The listing builds one solid part. Answer for the finished solid, in the listing's coordinates (mm). Face numbers are marked on the shaded views. A direction names the side the tool comes from. Coordinates: 2 decimals unless noted, no trailing zeros. Loops run counter-clockwise (first coordinate to the right, second up) from the corner with the lowest first, then second, coordinate; pieces in that order, holes last. Notation, with made-up numbers: (72, -29.5) -> (86, -29.5) arc R27 cw to (86, -7.5) -> close; hole circle Ø6 at (14.5, -36). An arc over 180 degrees is marked (long way). Answer in a Markdown table with one row per item.
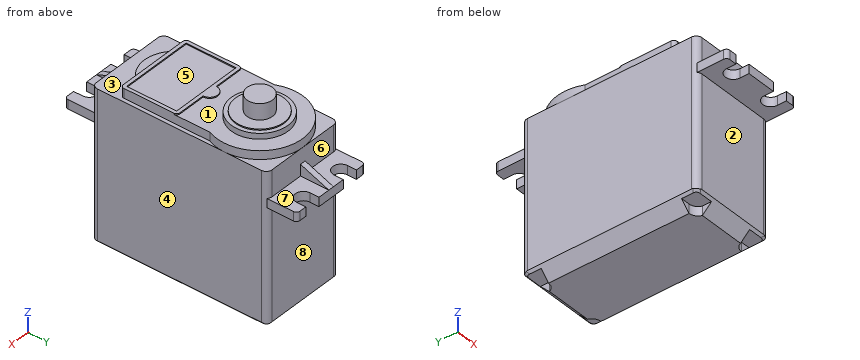
```python
from build123d import *

# Parameters (mm, degrees)
SKETCH1_W            = 35.433
SKETCH1_H            = 39.37
BOSS_EXTRUDE1_DEPTH  = 9.652
BOSS_EXTRUDE2_DEPTH  = 1.905
SKETCH3_R            = 6.35
BOSS_EXTRUDE3_DEPTH  = 1.27
SKETCH4_R            = 5.461
BOSS_EXTRUDE4_DEPTH  = 0.254
SKETCH6_R            = 2.8575
BOSS_EXTRUDE5_DEPTH  = 3.556
FILLET1_R            = 0.762
BOSS_EXTRUDE6_START  = 0.254
SKETCH7_W            = 16.129
SKETCH7_H            = 11.176
BOSS_EXTRUDE6_DEPTH  = 0.254
CHAMFER1_SIZE        = 2.54
FILLET3_R            = 1.27
FILLET4_R            = 1.27
CUT_EXTRUDE1_DEPTH   = 2.032
MIRROR2_COPY_1_DEPTH = 2.032
BOSS_EXTRUDE7_DEPTH  = 2.032
BOSS_EXTRUDE8_DEPTH  = 0.635


with BuildPart() as part:
    # Sketch1 → Boss-Extrude1 (new, symmetric)
    with BuildSketch(Plane(origin=(0, 0, 0), x_dir=(0, 0, -1), z_dir=(1, 0, 0))):
        Rectangle(SKETCH1_W, SKETCH1_H)
    extrude(amount=BOSS_EXTRUDE1_DEPTH, both=True)

    # Sketch2 → Boss-Extrude2 (add)
    with BuildSketch(Plane.XY.offset(17.7165)):
        with BuildLine():
            Line((-8.8265, 6.127362824), (-8.8265, -13.8938))
            Line((-8.8265, -13.8938), (-4.7625, -13.8938))
            ThreePointArc((-4.7625, -13.8938), (0, -15.817151304), (4.7625, -13.8938))
            Line((4.7625, -13.8938), (8.8265, -13.8938))
            Line((8.8265, -13.8938), (8.8265, 6.127362824))
            ThreePointArc((8.8265, 6.127362824), (0, 19.685), (-8.8265, 6.127362824))
        make_face()
    extrude(amount=BOSS_EXTRUDE2_DEPTH)

    # Sketch3 → Boss-Extrude3 (add)
    with BuildSketch(Plane.XY.offset(19.6215)):
        with Locations(Location((0, 10.033, 0), (0, 0, 180))):
            Circle(SKETCH3_R)
    extrude(amount=BOSS_EXTRUDE3_DEPTH)

    # Sketch4 → Boss-Extrude4 (add)
    with BuildSketch(Plane.XY.offset(20.8915)):
        with Locations((0, 10.033)):
            Circle(SKETCH4_R)
    extrude(amount=BOSS_EXTRUDE4_DEPTH)

    # Sketch6 → Boss-Extrude5 (add)
    with BuildSketch(Plane.XY.offset(21.1455)):
        with Locations((0, 10.033)):
            Circle(SKETCH6_R)
    extrude(amount=BOSS_EXTRUDE5_DEPTH)

    # Fillet1
    fillet1_edges = [part.edges().sort_by_distance(p)[0] for p in [
        (-8.8265, -13.8938, 18.669),
        (8.8265, -13.8938, 18.669),
    ]]
    fillet(fillet1_edges, radius=FILLET1_R)

    # Sketch7 → Boss-Extrude6 (add)
    with BuildSketch(Plane.XY.offset(19.6215).offset(BOSS_EXTRUDE6_START)):
        with BuildLine():
            Line((8.8265, -13.1318), (8.8265, -1.9558))
            ThreePointArc((8.8265, -1.9558), (8.603315367, -1.416984633), (8.0645, -1.1938))
            Line((8.0645, -1.1938), (1.778, -1.1938))
            ThreePointArc((1.778, -1.1938), (0, 0.5842), (-1.778, -1.1938))
            Line((-1.778, -1.1938), (-8.0645, -1.1938))
            ThreePointArc((-8.0645, -1.1938), (-8.603315367, -1.416984633), (-8.8265, -1.9558))
            Line((-8.8265, -1.9558), (-8.8265, -13.1318))
            ThreePointArc((-8.8265, -13.1318), (-8.603315367, -13.670615367), (-8.0645, -13.8938))
            Line((-8.0645, -13.8938), (8.0645, -13.8938))
            ThreePointArc((8.0645, -13.8938), (8.603315367, -13.670615367), (8.8265, -13.1318))
        make_face()
        with Locations((0, -7.5438)):
            Rectangle(SKETCH7_W, SKETCH7_H, mode=Mode.SUBTRACT)
    extrude(amount=-BOSS_EXTRUDE6_DEPTH)

    # Chamfer1
    chamfer1_edges = [part.edges().sort_by_distance(p)[0] for p in [
        (9.652, 0, -17.7165),
        (-9.652, 0, -17.7165),
        (0, 19.685, -17.7165),
        (0, -19.685, -17.7165),
    ]]
    chamfer(chamfer1_edges, length=CHAMFER1_SIZE)

    # Fillet3
    # the kernel refuses this fillet: 1.27 mm, written as the material it takes off along each edge
    with BuildSketch(Plane(origin=(9.652, 19.685, -18.3515), x_dir=(0, -1, 0), z_dir=(0, 0, 1))) as fillet3_piece_1:
        with BuildLine():
            CenterArc((FILLET3_R, -FILLET3_R), FILLET3_R, 90, 90)
            Line((0, -FILLET3_R), (0, 0))
            Line((0, 0), (FILLET3_R, 0))
        make_face()
    extrude(amount=39.243, mode=Mode.SUBTRACT)
    with BuildSketch(Plane(origin=(10.710333333, 20.743333333, -14.118166667), x_dir=(0.408248290463863, -0.816496580927726, 0.408248290463863), z_dir=(-0.5773502691896258, -0.5773502691896257, -0.5773502691896257))) as fillet3_piece_2:
        with BuildLine():
            CenterArc((FILLET3_R * 0.57735026919, FILLET3_R), FILLET3_R, 210, 60)
            Line((-FILLET3_R * 0.288675134595, FILLET3_R * 0.5), (0, 0))
            Line((0, 0), (FILLET3_R * 0.57735026919, 0))
        make_face()
    extrude(amount=8.065583261, mode=Mode.SUBTRACT)

    # Fillet4
    # the kernel refuses this fillet: 1.27 mm, written as the material it takes off along each edge
    with BuildSketch(Plane(origin=(-9.652, 19.685, -18.3515), x_dir=(0, -1, 0), z_dir=(0, 0, 1))) as fillet4_piece_1:
        with BuildLine():
            CenterArc((FILLET4_R, FILLET4_R), FILLET4_R, 180, 90)
            Line((0, FILLET4_R), (0, 0))
            Line((0, 0), (FILLET4_R, 0))
        make_face()
    extrude(amount=39.243, mode=Mode.SUBTRACT)
    with BuildSketch(Plane(origin=(-6.053666667, 16.086666667, -18.774833333), x_dir=(0.816496580927726, 0.40824829046386296, 0.40824829046386296), z_dir=(-0.5773502691896257, 0.5773502691896258, 0.5773502691896258)), Plane(origin=(10.710333333, -20.743333333, -14.118166667), x_dir=(0.4082482904638618, 0.816496580927726, 0.40824829046386424), z_dir=(-0.5773502691896258, 0.5773502691896257, -0.5773502691896257))) as fillet4_piece_2:
        with BuildLine():
            CenterArc((FILLET4_R * 0.57735026919, -FILLET4_R), FILLET4_R, 90, 60)
            Line((-FILLET4_R * 0.288675134595, -FILLET4_R * 0.5), (0, 0))
            Line((0, 0), (FILLET4_R * 0.57735026919, 0))
        make_face()
    extrude(amount=8.065583261, mode=Mode.SUBTRACT)
    with BuildSketch(Plane(origin=(-6.053666667, -16.086666667, -18.774833333), x_dir=(0.8164965809277258, -0.4082482904638633, 0.4082482904638633), z_dir=(-0.5773502691896261, -0.5773502691896256, 0.5773502691896256))) as fillet4_piece_3:
        with BuildLine():
            CenterArc((FILLET4_R * 0.57735026919, FILLET4_R), FILLET4_R, 210, 60)
            Line((-FILLET4_R * 0.288675134595, FILLET4_R * 0.5), (0, 0))
            Line((0, 0), (FILLET4_R * 0.57735026919, 0))
        make_face()
    extrude(amount=8.065583261, mode=Mode.SUBTRACT)
    with BuildSketch(Plane(origin=(-9.652, -19.685, 20.8915), x_dir=(1, 0, 0), z_dir=(0, 0, -1)), Plane(origin=(9.652, -19.685, 20.8915), x_dir=(0, 1, 0), z_dir=(0, 0, -1))) as fillet4_piece_4:
        with BuildLine():
            CenterArc((FILLET4_R, -FILLET4_R), FILLET4_R, 90, 90)
            Line((0, -FILLET4_R), (0, 0))
            Line((0, 0), (FILLET4_R, 0))
        make_face()
    extrude(amount=39.243, mode=Mode.SUBTRACT)

    # Sketch9 → Cut-Extrude1 (cut)
    with BuildSketch(Plane(origin=(0, 0, -17.7165), x_dir=(-1, 0, 0), z_dir=(0, 0, -1))):
        with BuildLine():
            Line((-5.181767112, 17.145), (-5.181767112, 19.685))
            Line((-5.181767112, 19.685), (-9.652, 19.685))
            Line((-9.652, 19.685), (-9.652, 15.748))
            Line((-9.652, 15.748), (-7.112, 15.748))
            ThreePointArc((-7.112, 15.748), (-5.920634397, 16.133891863), (-5.181767112, 17.145))
        make_face()
    cut_extrude1 = extrude(amount=-CUT_EXTRUDE1_DEPTH, mode=Mode.SUBTRACT)

    # Mirror1: Cut-Extrude1 across plane
    add(cut_extrude1.mirror(Plane.ZX), mode=Mode.SUBTRACT)

    # Mirror2: Cut-Extrude1 across plane
    add(cut_extrude1.mirror(Plane(origin=(0, 0, 0), x_dir=(0, 0, 1), z_dir=(1, 0, 0))), mode=Mode.SUBTRACT)

    # Mirror2 copy 1 sketch → Mirror2 copy 1 (cut)
    with BuildSketch(Plane(origin=(0, 0, -17.7165), x_dir=(1, 0, 0), z_dir=(0, 0, -1))):
        with BuildLine():
            Line((-5.181767112, 17.145), (-5.181767112, 19.685))
            Line((-5.181767112, 19.685), (-9.652, 19.685))
            Line((-9.652, 19.685), (-9.652, 15.748))
            Line((-9.652, 15.748), (-7.112, 15.748))
            ThreePointArc((-7.112, 15.748), (-5.920634397, 16.133891863), (-5.181767112, 17.145))
        make_face()
    extrude(amount=-MIRROR2_COPY_1_DEPTH, mode=Mode.SUBTRACT)

    # Sketch13 → Boss-Extrude7 (add)
    with BuildSketch(Plane.XY.offset(11.8745)):
        with BuildLine():
            Line((-9.280025612, -19.313025612), (-9.280025612, -25.273))
            ThreePointArc((-9.280025612, -25.273), (-9.056840979, -25.811815367), (-8.518025612, -26.035))
            Line((-8.518025612, -26.035), (-6.858, -26.035))
            Line((-6.858, -26.035), (-6.858, -24))
            ThreePointArc((-6.858, -24), (-5.08, -22.222), (-3.302, -24))
            Line((-3.302, -24), (-3.302, -26.035))
            Line((-3.302, -26.035), (3.302, -26.035))
            Line((3.302, -26.035), (3.302, -24))
            ThreePointArc((3.302, -24), (5.08, -22.222), (6.858, -24))
            Line((6.858, -24), (6.858, -26.035))
            Line((6.858, -26.035), (8.518025612, -26.035))
            ThreePointArc((8.518025612, -26.035), (9.056840979, -25.811815367), (9.280025612, -25.273))
            Line((9.280025612, -25.273), (9.280025612, -19.313025612))
            ThreePointArc((9.280025612, -19.313025612), (8.868007959, -19.588327006), (8.382, -19.685))
            Line((8.382, -19.685), (-8.382, -19.685))
            ThreePointArc((-8.382, -19.685), (-8.868007959, -19.588327006), (-9.280025612, -19.313025612))
        make_face()
    boss_extrude7 = extrude(amount=-BOSS_EXTRUDE7_DEPTH)

    # Sketch14 → Boss-Extrude8 (add, symmetric)
    with BuildSketch(Plane(origin=(0, 0, 0), x_dir=(0, 0, -1), z_dir=(1, 0, 0))):
        Polygon((-11.8745, -26.035), (-14.4145, -19.685), (-11.8745, -19.685), align=None)
    boss_extrude8 = extrude(amount=BOSS_EXTRUDE8_DEPTH, both=True)

    # Mirror3: Boss-Extrude7, Boss-Extrude8 across plane
    add(boss_extrude7.mirror(Plane.ZX))
    add(boss_extrude8.mirror(Plane.ZX))


solid = part.part
```
Item 1: A cutting plane is placed at D-D, the plane y = -5. Determine the outline of the cut face in (x, z), plus the area to 3 significant figures.
Findings below:
| item | result |
|---|---|
| outline | (-9.65, -15.18) -> (-7.11, -17.72) -> (7.11, -17.72) -> (9.65, -15.18) -> (9.65, 17.72) -> (8.83, 17.72) -> (8.83, 19.88) -> (8.06, 19.88) -> (8.06, 19.62) -> (-8.06, 19.62) -> (-8.06, 19.88) -> (-8.83, 19.88) -> (-8.83, 17.72) -> (-9.65, 17.72) -> close |
| area | 712 mm2 |
Item 2: A tool of negligible diameter and unlimited length cuts with its end or side. For the marked faces 4, 5, 6, 7 and 8, from which of +Z, -Z, +X, -X, +Y, -Y can it reach the whole face along a straight path? Write none if from no direction.
Findings below:
| item | result |
|---|---|
| face 4 | +Z, -Z, +X, +Y, -Y |
| face 5 | +Z |
| face 6 | +Z, +Y |
| face 7 | +Z, +X, +Y |
| face 8 | -Z, +X, -X, +Y |
Item 3: A cutting plane is placed at A-A, the plane y = 2.5. Determine the outline of the cut face in (x, z).
Findings below:
| item | result |
|---|---|
| outline | (-9.65, -15.18) -> (-7.11, -17.72) -> (7.11, -17.72) -> (9.65, -15.18) -> (9.65, 17.72) -> (8.83, 17.72) -> (8.83, 19.62) -> (-8.83, 19.62) -> (-8.83, 17.72) -> (-9.65, 17.72) -> close |
Item 4: Determine the mould class of the marked faces 1, 2 and 3 for opening direction Y: +Y half, -Y half, draft (parallel to the pull), parting line (faces both ways), or undercut.
Findings below:
| item | result |
|---|---|
| face 1 | undercut |
| face 2 | -Y half |
| face 3 | draft |
Item 5: Find the intervals of material crossed by probe 1 along Z at (x, y) = (-2, 23); probe 2 along Y at (x, z) = (-5, -1.5) (3 decimals); probe 3 along Z at (x, y) = (-7.5, -17.5), in increasing order.
Findings below:
| item | result |
|---|---|
| probe 1 | z = 9.84 to 11.87 |
| probe 2 | y = -19.685 to 19.685 |
| probe 3 | z = -15.68 to 17.72 |
Item 6: A cutting plane is placed at B-B, the plane z = -8. Determine the outline of the cut face in (x, y) (3 decimals).
Findings below:
| item | result |
|---|---|
| outline | (-9.652, -18.415) arc R1.27 ccw to (-8.382, -19.685) -> (8.382, -19.685) arc R1.27 ccw to (9.652, -18.415) -> (9.652, 18.415) arc R1.27 ccw to (8.382, 19.685) -> (-8.382, 19.685) arc R1.27 ccw to (-9.652, 18.415) -> close |
Item 7: Flat-ended cylindrical pins translate along their axes: pin 1 Ø1 at (y, z) = (25, 11) entering from -X; pin 2 Ø1.5 at (x, z) = (3, 4.5) entering from +Y (3 decimals); pin 3 Ø3.5 at (x, y) = (0.5, -22) entering from -Z. Find the tip coordinate at first contact, or state that the pin passes through.
Findings below:
| item | result |
|---|---|
| pin 1 | stops at x = -9.28 |
| pin 2 | stops at y = 19.685 |
| pin 3 | stops at z = 9.84 |
